Check sheet for the modelled part. Datum: model origin and axes. Units: mm. A direction names the side the tool comes from. Coordinates: 2 decimals unless noted, no trailing zeros. Write each question's results on one line, items separated by ' | '. Start each with the question number.
1. Gauge pin test, flat ends, axial feed: P1, Ø10, axis at x = -35.5, z = 7.5, coming from the +Y side; P2, Ø2, axis at y = -4.5, z = 3, coming from the +X side; P3, Ø1, axis at y = -2, z = 31, coming from the +X side. Record the tip position at first contact, or that the pin passes through.
2. Tool access check on faces 1 (the face through (-40.588, -1.833, 2.897)), 2 (the face through (5.54, 0.296, 49.673)). Record the directions out of +Z, -Z, +X, -X, +Y, -Y that give a thin tool (end or side, any length) a straight path to the whole face; none if there is none.
3. Thickness scan on line 1 (Y direction, x = -24, z = -1); line 2 (Y direction, x = 11, z = 1); line 3 (Z direction, x = 10, y = -5.5). Record the ranges inside material, lowest first. Write a range as [from, to].
```python
from build123d import *

# Parameters (mm, degrees)
F1_DEPTH = 6.1
F2_R     = 6.096
F3_R     = 4.18
F4_DEPTH = 0.6


with BuildPart() as f1:
    # F0 (on Front) → F1 (new body)
    with BuildSketch(Plane.XZ):
        with BuildLine():
            Line((8.623609, 65.353912), (-34.706391, 65.353912))
            ThreePointArc((-34.706391, 65.353912), (-40.094544, 63.122066), (-42.326391, 57.733912))
            Line((-42.326391, 57.733912), (-42.326391, -50.426088))
            ThreePointArc((-42.326391, -50.426088), (-40.094544, -55.814242), (-34.706391, -58.046088))
            Line((-34.706391, -58.046088), (8.623609, -58.046088))
            ThreePointArc((8.623609, -58.046088), (14.011763, -55.814242), (16.243609, -50.426088))
            Line((16.243609, -50.426088), (16.243609, 57.733912))
            ThreePointArc((16.243609, 57.733912), (14.011763, 63.122066), (8.623609, 65.353912))
        make_face()
    extrude(amount=F1_DEPTH)

    # F2
    f2_edges = [f1.edges().sort_by_distance(p)[0] for p in [
        (16.243609, 0, 3.653912),
        (14.011763, 0, 63.122066),
        (-13.041391, 0, 65.353912),
        (-40.094544, 0, 63.122066),
        (-42.326391, 0, 3.653912),
        (-40.094544, 0, -55.814242),
        (-13.041391, 0, -58.046088),
        (14.011763, 0, -55.814242),
    ]]
    fillet(f2_edges, radius=F2_R)

    # F3 (on face) → F4 (join)
    with BuildSketch(Plane(origin=(0, 0, 0), x_dir=(-1, 0, 0), z_dir=(0, 1, 0))):
        with Locations((-4.633609, 53.753912)):
            Circle(F3_R)
    extrude(amount=F4_DEPTH)


solid = f1.part
```
Established:
1) P1: y = 0 | P2: x = 16.21 | P3: x = 15.07
2) face 1: +Z, -Z, -X, +Y | face 2: +Y
3) line 1: [-6.1, 0] | line 2: [-6.1, -0.06] | line 3: [-57.89, 65.2]
